Could you check a few things on this model? Use its own coordinates, in mm. A direction names the side the tool comes from. Coordinates: 2 decimals unless noted, no trailing zeros. Order: outer loops, then holes, each group sorted by start corner. A loop starts at its lowest first (then second) coordinate and runs counter-clockwise, first axis right, second up. Notation, with made-up numbers: M 2.5,40.5 L 59.5,40.5 A13 cw 59.5,64.5 Z; hole C 76.5,-3.75 d9. An arc over 180 degrees is marked long. Put each result on its own line as item: value. Start each with the question number.
```python
from build123d import *

# Parameters (mm, degrees)
F2_SIZE = 0.2
F3_R    = 1


with BuildPart() as f1:
    # F0 (on Top) → F1 (revolve)
    with BuildSketch(Plane.XY):
        Polygon((2.5, 6), (2.5, 0), (4, 0), (4, 7), (5.75, 7), (5.75, 7.5), (10.75, 7.5), (10.75, 9), (0, 9), (0, 6), align=None)
    revolve(axis=Axis((0, 5.832618, 0), (0, -1, 0)))

    # F2
    f2_edges = [f1.edges().sort_by_distance(p)[0] for p in [
        (-4, 0, 0),
    ]]
    chamfer(f2_edges, length=F2_SIZE)

    # F3
    f3_edges = [f1.edges().sort_by_distance(p)[0] for p in [
        (-10.75, 9, 0),
    ]]
    fillet(f3_edges, radius=F3_R)


solid = f1.part
```
Item 1: I need wall thicknesses on probe 1 along Z at (x, y) = (0, 1.3); probe 2 along Y at (x, z) = (-3.75, -3); probe 3 along Y at (x, z) = (-4, 5.5). Which ranges of each line are inside material? Lowest first, please.
Item 2: For faces 1 (the flat face through (0, 9, 0)), 2 (the cylindrical face through (-0.867, 3.648, -3.905)), which set-ups out of +Z, -Z, +X, -X, +Y, -Y let a thin tool reach every point of the face, with its end or its side?
Item 3: For pin 1 Ø1.5 at (x, z) = (0, 0.5) entering from -Y, with a flat end and sliding along its axis, tell me the tip position at first contact or that it passes through.
Item 4: If we section it at A-A on z = 0: Write out the boundary of the cut face in (x, y).
Item 5: If we mould it in two halves opening along X, with no side actions, what happens to faces 3 (the flat face through (0, 6, 0)), 4 (the flat face through (-2, 7, -4)), 5 (the cylindrical face through (-0.75, 7.25, 5.7))? For each: released by +X, released by -X, zero draft, split by the parting line, or undercut.
Item 6: If we section it at C-C on y = 5.5: Write out the boundary of the cut face in (x, z), then the cut area to 3 significant figures.
Item 7: If we section it at B-B on x = 0: Write out the boundary of the cut face in (y, z), then the cut area to 3 significant figures.
Geometry check:
1. probe 1: z = -4 to -2.5, 2.5 to 4
1. probe 2: y = 7 to 9
1. probe 3: y = 7.5 to 9
2. face 1: +Z, -Z, +X, -X, +Y
2. face 2: -Y
3. pin 1: stops at y = 6
4. outline: M -10.75,7.5 L -5.75,7.5 L -5.75,7 L -4,7 L -4,0.2 L -3.8,0 L -2.5,0 L -2.5,6 L 2.5,6 L 2.5,0 L 3.8,0 L 4,0.2 L 4,7 L 5.75,7 L 5.75,7.5 L 10.75,7.5 L 10.75,8 A1 ccw 9.75,9 L -9.75,9 A1 ccw -10.75,8 Z
5. face 3: undercut
5. face 4: zero draft
5. face 5: split by the parting line
6. outline: C 0,0 d8; hole C 0,0 d5
6. area: 30.6 mm²
7. outline: M 0,-3.8 L 0.2,-4 L 7,-4 L 7,-5.75 L 7.5,-5.75 L 7.5,-10.75 L 8,-10.75 A1 ccw 9,-9.75 L 9,9.75 A1 ccw 8,10.75 L 7.5,10.75 L 7.5,5.75 L 7,5.75 L 7,4 L 0.2,4 L 0,3.8 L 0,2.5 L 6,2.5 L 6,-2.5 L 0,-2.5 Z
7. area: 63.5 mm²
